Autodesk Inventor part; units mm, degrees
ref_plane "YZ Plane" through (0, 0, 0) normal (1, 0, 0) x (0, 1, 0)
ref_plane "XZ Plane" through (0, 0, 0) normal (0, 1, 0) x (-1, 0, 0)
ref_plane "XY Plane" through (0, 0, 0) normal (0, 0, 1) x (1, 0, 0)
sketch "Szkic1" plane through (0, 0, 0) normal (0, 0, 1) x (1, 0, 0)
  line L0 (-28.7, 0) -> (28.7, 0) construction
  line L1 (0, -17.36) -> (0, 17.36) construction
  line L2 (-20.5, -12.4) -> (20.5, -12.4)
  line L3 (20.5, -12.4) -> (20.5, 12.4)
  line L4 (20.5, 12.4) -> (-20.5, 12.4)
  line L5 (-20.5, 12.4) -> (-20.5, -12.4)
  line L6 (-20.5, -12.4) -> (20.5, 12.4) construction
  line L7 (20.5, -12.4) -> (-20.5, 12.4) construction
  point P0 (0, 0)
  dimension "d0" = 41
  dimension "d1" = 24.8
extrude "Wyciągnięcie proste1" add sketch "Szkic1" along normal blind 10
sketch "Szkic2" plane through (-20.5, -12.4, 0) normal (0, -1, 0) x (1, 0, 0)
  point P0 (20.5, 0)
sketch "Szkic3" plane through (-20.5, -12.4, 0) normal (0, -1, 0) x (1, 0, 0)
  line L0 (-8.2, 0) -> (49.2, 0) construction
  line L1 (20.5, -2) -> (20.5, 12) construction
  line L2 (5.5, 6) -> (5.5, 0)
  line L3 (0, 0) -> (41, 0)
  line L4 (5.5, 6) -> (7.5, 6)
  line L5 (7.5, 6) -> (7.5, 2)
  line L6 (7.5, 2) -> (11.5, 2) construction
  line L7 (11.5, 2) -> (11.5, 6)
  line L8 (11.5, 6) -> (13.5, 6)
  line L9 (13.5, 6) -> (13.5, 0)
  line L10 (5.5, 0) -> (13.5, 0)
  line L11 (0, 0) -> (0, 10)
  line L12 (0, 0) -> (41, 0)
  line L13 (41, 0) -> (41, 10)
  line L14 (41, 10) -> (0, 10)
  line L15 (0, 10) -> (0, 0)
  arc A0 (7.5, 2) -> (11.5, 2) centre (9.5, 3.8138) ccw
  line L16 (35.5, 6) -> (35.5, 0)
  line L17 (35.5, 6) -> (33.5, 6)
  line L18 (33.5, 6) -> (33.5, 2)
  line L19 (29.5, 2) -> (29.5, 6)
  line L20 (29.5, 6) -> (27.5, 6)
  line L21 (27.5, 6) -> (27.5, 0)
  arc A1 (29.5, 2) -> (33.5, 2) centre (31.5, 3.8138) ccw
  circle A2 centre (31.5, 2.8) radius 1.6
  circle A3 centre (9.5, 2.8) radius 1.6
  point P0 (20.5, 0)
  point P1 (20.5, 0)
  dimension "d4" = 6
  dimension "d5" = 15
  dimension "d6" = 2
  dimension "d7" = 4
  dimension "d8" = 4
  dimension "d9" = 4
  dimension "d10" = 2
  dimension "d11" = 20.5
  dimension "d12" = 10
  dimension "d13" = 2.7
  dimension "d16" = 3.2
  dimension "d17" = 2.8
  dimension "d18" = 11
extrude "Wyciągnięcie proste2" add sketch "Szkic3" along normal blind 2 and the other way blind 27 contours L2 L3 L11 L14 L13 L16 L17 L18 A1 L19 L20 L21 L9 L8 L7 A0 L5 L4 | A2 | A3
extrude "Wyciągnięcie proste3" cut sketch "Szkic3" along normal through all both and the other way through all contours A2 | A3
properties part number "uMule-uchwyt_dx"
Geometry check sheet. Reference: the model listing, model coordinates, mm. A direction names the side the tool comes from. Coordinates: 2 decimals unless noted, no trailing zeros. Write each loop counter-clockwise with the first axis right and the second up, starting at its lowest first coordinate (ties: lowest second). Pieces come first, ordered by that corner, then holes. Notation, with made-up numbers: M 68.25,2.25 L 77.25,2.25 A22 ccw 77.25,30.25 Z; hole C 33.25,63.25 d11. An arc over 180 degrees is marked long. Answer as a JSON object with one key per item and string values.
1. Scan lines: L1, parallel to X at y = 1.75, z = 2.8; L2, parallel to Z at x = -11, y = -1; L3, parallel to X at y = -2.25, z = 3.75. Record each from-to range of solid material in increasing order.
Answers below:
{"L1": "x = -20.5 to -12.6, -9.4 to 9.4, 12.6 to 20.5", "L2": "z = 0 to 1.2, 4.4 to 10", "L3": "x = -20.5 to -12.29, -9.71 to 9.71, 12.29 to 20.5"}
2. Section check C-C, the plane z = 2.8. Give the number of separate pieces and of enclosed holes in the cut face, plus the area to 3 significant figures.
Answers below:
{"separate pieces": "3", "enclosed holes": "0", "area": "970 mm²"}
3. Tool access check on faces 4 (the flat face through (11.06, 12.4, 0.96)), 5 (the flat face through (7, -13, 3)), 6 (the cylindrical face through (-12.6, -0.1, 2.87)). Record the directions out of +Z, -Z, +X, -X, +Y, -Y that give a thin tool (end or side, any length) a straight path to the whole face; none if there is none.
Answers below:
{"face 4": "-Z, +Y", "face 5": "-Z, -Y", "face 6": "+Y, -Y"}
4. Go/stop test with flat-tipped pins: pin 1 Ø3 at (x, y) = (14.5, 8) entering from -Z; pin 2 Ø1.6 at (x, y) = (-14, 14) entering from -Z. Record where each tip stops, or that it passes through.
Answers below:
{"pin 1": "stops at z = 0", "pin 2": "stops at z = 6"}
5. Section check A-A, the plane x = -11. Enter the section's corners in (y, z), plus the area to 3 significant figures.
Answers below:
{"outline": "M -14.4,1.11 L -12.4,1.11 L -12.4,0 L 12.4,0 L 12.4,1.11 L 14.6,1.11 L 14.6,1.2 L -14.4,1.2 Z; M -14.4,4.4 L 14.6,4.4 L 14.6,10 L -14.4,10 Z", "area": "193 mm²"}
6. Draft check along X on faces 1 (the flat face through (-14, -13, 6)), 2 (the flat face through (0, -14.4, 6)), 3 (the flat face through (20.5, 0, 5)). Enter one of: released by +X, released by -X, zero draft, split by the parting line, or undercut.
Answers below:
{"face 1": "undercut", "face 2": "zero draft", "face 3": "released by +X"}
7. Section check B-B, the plane y = 11.5. Enter the section's corners in (x, z), plus the area to 3 significant figures.
Answers below:
{"outline": "M -20.5,0 L 20.5,0 L 20.5,10 L -20.5,10 Z; hole C -11,2.8 d3.2; hole C 11,2.8 d3.2", "area": "394 mm²"}
